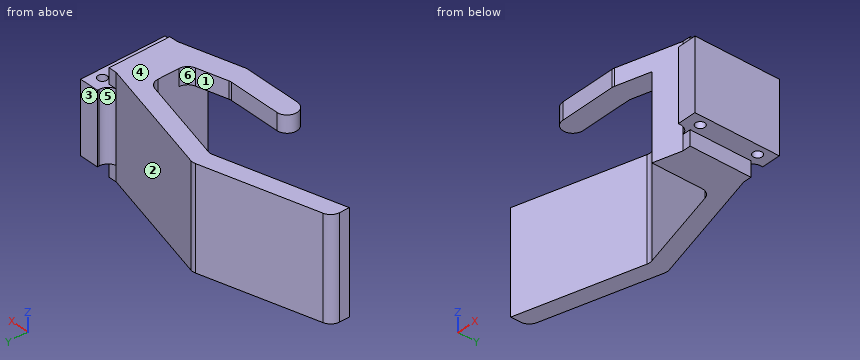
Autodesk Inventor part; units mm, degrees
ref_plane "YZ Plane" through (0, 0, 0) normal (1, 0, 0) x (0, 1, 0)
ref_plane "XZ Plane" through (0, 0, 0) normal (0, 1, 0) x (-1, 0, 0)
ref_plane "XY Plane" through (0, 0, 0) normal (0, 0, 1) x (1, 0, 0)
sketch "Sketch1" plane through (0, 0, 0) normal (0, 0, 1) x (1, 0, 0)
  line L0 (52.1089, 41.9337) -> (16.0623, 32.275)
  line L1 (81.0151, 18.2189) -> (81.0151, 29.0119)
  line L2 (81.0151, 29.0119) -> (52.1089, 36.7573)
  line L3 (52.1089, 36.7573) -> (16.0623, 27.0986)
  line L4 (16.0623, 32.275) -> (16.0623, 27.0986)
  line L5 (71.0038, 9.1932) -> (89.0623, 14.032)
  line L6 (71.0038, 9.1932) -> (54.0038, 9.1932)
  line L7 (54.0092, 15.1932) -> (69.7233, 15.1932)
  arc A0 (54.0092, 15.1932) -> (54.0038, 9.1932) centre (54.0065, 12.1932) ccw
  line L8 (69.7233, 15.1932) -> (81.0151, 18.2189)
  line L9 (52.1089, 41.9337) -> (89.0623, 32.032)
  line L10 (97.0623, 35.532) -> (97.0623, 10.532)
  circle A1 centre (94.2623, 31.5608) radius 1.35
  circle A2 centre (94.2623, 14.5608) radius 1.35
  line L11 (89.0623, 32.032) -> (91.4623, 32.032)
  line L12 (91.4623, 32.032) -> (91.4623, 35.532)
  line L13 (91.4623, 35.532) -> (97.0623, 35.532)
  line L14 (89.0623, 14.032) -> (91.4623, 14.032)
  line L15 (91.4623, 14.032) -> (91.4623, 10.532)
  line L16 (91.4623, 10.532) -> (97.0623, 10.532)
  point P0 (0, 0)
  dimension "d0" = 5
  dimension "d1" = 6
  dimension "d2" = 5
  dimension "d3" = 75
  dimension "d4" = 150
  dimension "d5" = 18
  dimension "d6" = 15
  dimension "d28" = 25
  dimension "d30" = 5.6
  dimension "d31" = 5.6
extrude "Extrusion1" add sketch "Sketch1" along normal blind 30
sketch "Sketch3" plane through (0, 0, 0) normal (0, 0, -1) x (-1, 0, 0)
  line L0 (-81.0151, 18.2189) -> (-46.6558, 18.2189)
  line L1 (-46.6558, 18.2189) -> (-46.6558, 4.635)
  line L2 (-46.6558, 4.635) -> (-81.0151, 4.635)
  line L3 (-81.0151, 4.635) -> (-81.0151, 18.2189)
  point P0 (0, 0)
extrude "Extrusion2" cut sketch "Sketch3" against normal blind 25
fillet "Fillet1" radius 3 7 edges at (81.0151, 29.0119, 15) (81.0151, 18.2189, 27.5) (69.7233, 15.1932, 27.5) (52.1089, 36.7573, 15) (52.1089, 41.9337, 15) (16.0623, 32.275, 15) (71.0038, 9.1932, 27.5)
sketch "Sketch6" plane through (91.4623, 35.532, 0) normal (0, 1, 0) x (1, 0, 0)
  line L0 (0, 0) -> (0, -30)
  line L1 (5.6, 0) -> (0, 0)
  line L2 (0, 0) -> (0, -4.5)
  line L3 (0, -4.5) -> (5.6, -4.5)
  line L4 (5.6, -4.5) -> (5.6, 0)
  line L5 (5.6, -30) -> (0, -30)
  line L6 (0, -30) -> (0, -25.5)
  line L7 (0, -25.5) -> (5.6, -25.5)
  line L8 (5.6, -25.5) -> (5.6, -30)
  point P0 (-91.4623, 0)
  dimension "d32" = 4.5
  dimension "d33" = 5.6
  dimension "d34" = 4.5
extrude "Extrusion5" cut sketch "Sketch6" against normal through all
fillet "Fillet2" radius 3 2 edges at (91.4623, 32.032, 15) (91.4623, 14.032, 15)
properties part number "Right Hand" material "Aluminum-6061"
Geometry check sheet. Reference: the model listing, model coordinates, mm. Face numbers are marked on the shaded views. A direction names the side the tool comes from. Coordinates: 2 decimals unless noted, no trailing zeros. Loops run counter-clockwise (first coordinate to the right, second up) from the corner with the lowest first, then second, coordinate; pieces in that order, holes last. Notation, with made-up numbers: (28.25, 6.5) - (43.25, 6.5) arc R19 ccw to (43.25, 16.5) - close; hole circle Ø6 at (-23.5, -25.5). An arc over 180 degrees is marked (long way). One line per item, written item: value. Start each with the question number.
(1) Mould release check, pull along Y, two halves, no side actions. Record for the marked faces 4, 5 and 6: released by +Y, released by -Y, zero draft, split by the parting line, or undercut.
(2) Material ranges on line 1 (X direction, y = 21, z = 13.5); line 2 (Z direction, x = 58.5, y = 13); line 3 (Y direction, x = 65, z = 26.5), recorded low to high. Write a range as [from, to].
(3) Cross-section at A-A on y = 24. Enter the section's corners in (x, z), plus the area to 3 significant figures.
(4) Cross-section at B-B on x = 63.5. Enter the section's corners in (y, z).
(5) Cross-section at C-C on z = 3.25. Enter the section's corners in (x, y), plus the area to 3 significant figures.
(6) Depth check by flat-ended pin: P1, Ø1.6, axis at x = 94.26, y = 14.56, coming from the -Z side; P2, Ø4.5, axis at x = 95, z = 15, coming from the -Y side; P3, Ø6, axis at y = 17.5, z = 18.5, coming from the -X side; P4, Ø9, axis at x = 73.5, y = 16, coming from the -Z side. Enter the tip coordinate at first touch or a pass-through.
(7) Tool access check on the marked faces 1, 2 and 3. Record the directions out of +Z, -Z, +X, -X, +Y, -Y that give a thin tool (end or side, any length) a straight path to the whole face; none if there is none.
(8) Cross-section at D-D on z = 19. Enter the section's corners in (x, y).
Results below:
1. face 4: zero draft
1. face 5: released by +Y
1. face 6: undercut
2. line 1: x = [81.02, 97.06]
2. line 2: z = [25, 30]
2. line 3: y = [9.19, 15.19], [33.3, 38.48]
3. outline: (81.02, 0) - (91.46, 0) - (91.46, 4.5) - (97.06, 4.5) - (97.06, 25.5) - (91.46, 25.5) - (91.46, 30) - (81.02, 30) - close
3. area: 431 mm2
4. outline: (9.19, 25) - (15.19, 25) - (15.19, 30) - (9.19, 30) - close; (33.71, 0) - (38.88, 0) - (38.88, 30) - (33.71, 30) - close
5. outline: (16.06, 27.1) - (51.33, 36.55) arc R3 cw to (52.89, 36.55) - (78.79, 29.61) arc R3 cw to (81.02, 26.71) - (81.02, 11.88) - (89.06, 14.03) - (91.46, 14.03) - (91.46, 32.03) - (89.06, 32.03) - (52.89, 41.73) arc R3 ccw to (51.33, 41.73) - (18.29, 32.87) arc R3 ccw to (16.06, 29.97) - close
5. area: 542 mm2
6. P1: passes through
6. P2: stops at y = 10.53
6. P3: stops at x = 81.02
6. P4: stops at z = 25
7. face 1: +Z, -Z, -X
7. face 2: +Z, -Z, +Y
7. face 3: +Z, -Z, +X, +Y
8. outline: (16.06, 27.1) - (51.33, 36.55) arc R3 cw to (52.89, 36.55) - (78.79, 29.61) arc R3 cw to (81.02, 26.71) - (81.02, 11.88) - (89.06, 14.03) arc R3 cw to (91.46, 11.09) - (91.46, 10.53) - (97.06, 10.53) - (97.06, 35.53) - (91.46, 35.53) - (91.46, 34.97) arc R3 cw to (89.06, 32.03) - (52.89, 41.73) arc R3 ccw to (51.33, 41.73) - (18.29, 32.87) arc R3 ccw to (16.06, 29.97) - close; hole circle Ø2.7 at (94.26, 14.56); hole circle Ø2.7 at (94.26, 31.56)
